```python
from build123d import *

# Parameters (mm, degrees)
F1_DEPTH       = 12.7
F25_DEPTH      = 38.1
F3_D           = 3.175
F3_DEPTH       = 63.5
F3_CBORE_D     = 12.7
F3_CBORE_DEPTH = 6.35
F3_TIP         = 0.9538662327
F5_D           = 3.175
F5_DEPTH       = 63.5
F5_CBORE_D     = 12.7
F5_CBORE_DEPTH = 6.35
F5_TIP         = 0.9538662327
F7_D           = 3.175
F7_DEPTH       = 63.5
F7_TIP         = 0.9538662327
F9_D           = 3.175
F9_DEPTH       = 63.5
F9_TIP         = 0.9538662327
F10_W          = 330.2
F10_H          = 25.4
F11_DEPTH      = 6.35
F12_W          = 426.9362986088
F12_H          = 25.4
F13_DEPTH      = 6.35
F14_W          = 25.4
F14_H          = 558.8
F15_DEPTH      = 3.175
F16_W          = 25.4
F16_H          = 558.8
F17_DEPTH      = 3.175
F19_W          = 12.7
F19_H          = 25.4
F20_DEPTH      = 25.4
F18_W          = 165.1
F18_H          = 25.4
F21_DEPTH      = 3.175
F22_W          = 165.1
F22_H          = 25.4
F23_DEPTH      = 3.175


with BuildPart() as f1:
    # F0 (on Front) → F1 (new body, symmetric)
    with BuildSketch(Plane.XZ):
        with BuildLine():
            Line((165.1, 1828.8), (0, 1828.8))
            Line((0, 1828.8), (-165.1, 1828.8))
            Line((-165.1, 1828.8), (-165.1, 685.8))
            ThreePointArc((-165.1, 685.8), (-187.4175900274, 340.0309838924), (-254, 0))
            Line((-254, 0), (0, 0))
            Line((0, 0), (254, 0))
            ThreePointArc((254, 0), (187.4175900273, 340.0309838924), (165.1, 685.8))
            Line((165.1, 685.8), (165.1, 1828.8))
        make_face()
    extrude(amount=F1_DEPTH, both=True)

    # F24 (on face) → F25 (cut)
    with BuildSketch(Plane.XZ.offset(12.7)):
        Polygon((-12.7, 558.8), (0, 558.8), (12.7, 558.8), (12.7, 1828.8), (0, 1828.8), (-12.7, 1828.8), align=None)
    extrude(amount=-F25_DEPTH, mode=Mode.SUBTRACT)

    # F3
    with Locations(Plane.XZ.offset(12.7)):
        with Locations((-88.9, 1371.6), (88.9, 1371.6)):
            CounterBoreHole(F3_D / 2, F3_CBORE_D / 2, F3_CBORE_DEPTH, depth=F3_DEPTH)
            with Locations((0, 0, -(F3_DEPTH + F3_TIP / 2))):  # 118° drill point
                Cone(0, F3_D / 2, F3_TIP, mode=Mode.SUBTRACT)

    # F5
    with Locations(Plane(origin=(0, 12.7, 0), x_dir=(-1, 0, 0), z_dir=(0, 1, 0))):
        with Locations((-88.9, 457.2), (88.9, 457.2)):
            CounterBoreHole(F5_D / 2, F5_CBORE_D / 2, F5_CBORE_DEPTH, depth=F5_DEPTH)
            with Locations((0, 0, -(F5_DEPTH + F5_TIP / 2))):  # 118° drill point
                Cone(0, F5_D / 2, F5_TIP, mode=Mode.SUBTRACT)

    # F7
    with Locations(Plane.XY.offset(1828.8)):
        with Locations((-127, 0), (127, 0)):
            Hole(F7_D / 2, depth=F7_DEPTH)
            with Locations((0, 0, -(F7_DEPTH + F7_TIP / 2))):  # 118° drill point
                Cone(0, F7_D / 2, F7_TIP, mode=Mode.SUBTRACT)

    # F9
    with Locations(Plane(origin=(0, 0, 0), x_dir=(1, 0, 0), z_dir=(0, 0, -1))):
        with Locations((-190.5, 0), (190.5, 0)):
            Hole(F9_D / 2, depth=F9_DEPTH)
            with Locations((0, 0, -(F9_DEPTH + F9_TIP / 2))):  # 118° drill point
                Cone(0, F9_D / 2, F9_TIP, mode=Mode.SUBTRACT)

    # F10 (on face) → F11 (cut)
    with BuildSketch(Plane(origin=(0, 12.7, 0), x_dir=(-1, 0, 0), z_dir=(0, 1, 0))):
        with Locations((0, 1371.6)):
            Rectangle(F10_W, F10_H)
    extrude(amount=-F11_DEPTH, mode=Mode.SUBTRACT)

    # F12 (on face) → F13 (cut)
    with BuildSketch(Plane.XZ.offset(12.7)):
        with Locations((0, 457.2)):
            Rectangle(F12_W, F12_H)
    extrude(amount=-F13_DEPTH, mode=Mode.SUBTRACT)

    # F14 (on face) → F15 (cut)
    with BuildSketch(Plane(origin=(0, 12.7, 0), x_dir=(-1, 0, 0), z_dir=(0, 1, 0))):
        with Locations((0, 279.4)):
            Rectangle(F14_W, F14_H)
    extrude(amount=-F15_DEPTH, mode=Mode.SUBTRACT)

    # F16 (on face) → F17 (cut)
    with BuildSketch(Plane.XZ.offset(12.7)):
        with Locations((0, 279.4)):
            Rectangle(F16_W, F16_H)
    extrude(amount=-F17_DEPTH, mode=Mode.SUBTRACT)

    # F19 (on face) → F20 (cut)
    with BuildSketch(Plane.XZ.offset(12.7)):
        with Locations((165.1, 914.4)):
            Rectangle(F19_W, F19_H)
    extrude(amount=-F20_DEPTH, mode=Mode.SUBTRACT)

    # F18 (on face) → F21 (cut)
    with BuildSketch(Plane.XZ.offset(12.7)):
        with Locations((82.55, 914.4)):
            Rectangle(F18_W, F18_H)
    extrude(amount=-F21_DEPTH, mode=Mode.SUBTRACT)

    # F22 (on face) → F23 (cut)
    with BuildSketch(Plane(origin=(0, 12.7, 0), x_dir=(-1, 0, 0), z_dir=(0, 1, 0))):
        with Locations((-82.55, 914.4)):
            Rectangle(F22_W, F22_H)
    extrude(amount=-F23_DEPTH, mode=Mode.SUBTRACT)


solid = f1.part
```
The listing builds one solid part. Answer for the finished solid, in the listing's coordinates (mm). Give positions to 0.01 mm unless a question says otherwise; leave off trailing zeros. Write each loop counter-clockwise with the first axis right and the second up, starting at its lowest first coordinate (ties: lowest second). Pieces come first, ordered by that corner, then holes. Notation, with made-up numbers: (-27, 36.5) -> (-16, 36.5) arc R20 ccw to (-16, 75.5) -> close; hole circle Ø10 at (-34.5, 13). An arc over 180 degrees is marked (long way). Write item = value, one per line. Start each with the question number.
1) Each of these flat-tipped pins is pushed along its axis until it touches: pin 1 (6 mm diameter, centred on y = -5.5, z = 1001.5, fed in from -X); pin 2 (6.5 mm diameter, centred on x = -89, z = 460, fed in from +Y); pin 3 (7.5 mm diameter, centred on y = 6, z = 1364, fed in from +X). Where does it stop, or does it pass through?
2) The part is cut by section A-A, the plane z = 980. Determine the outline of the cut face in (x, y), and give its area (3 significant figures).
3) The part is cut by section B-B, the plane z = 178. Determine the outline of the cut face in (x, y) (3 decimals), and give its area (3 significant figures).
4) Straight lines are drawn through the part: line 1 along Z through (x, y) = (88.9, 9.25); line 2 along X through (y, z) = (0, 1809.5); line 3 along X through (y, z) = (-9, 1371.6). For each, find the intervals that lie inside material, in ascending order.
Solutions:
q1.pin_1 = -165.1
q1.pin_2 = 6.35
q1.pin_3 = 165.1
q2.outline = (-165.1, -12.7) -> (-12.7, -12.7) -> (-12.7, 12.7) -> (-165.1, 12.7) -> close; (12.7, -12.7) -> (165.1, -12.7) -> (165.1, 12.7) -> (12.7, 12.7) -> close
q2.area = 7,740 mm²
q3.outline = (-213.47, -12.7) -> (-12.7, -12.7) -> (-12.7, -9.525) -> (12.7, -9.525) -> (12.7, -12.7) -> (213.47, -12.7) -> (213.47, 12.7) -> (12.7, 12.7) -> (12.7, 9.525) -> (-12.7, 9.525) -> (-12.7, 12.7) -> (-213.47, 12.7) -> close
q3.area = 10,700 mm²
q4.line_1 = 0 to 450.85, 463.55 to 1358.9, 1384.3 to 1828.8
q4.line_2 = -165.1 to -128.59, -125.41 to -12.7, 12.7 to 125.41, 128.59 to 165.1
q4.line_3 = -165.1 to -95.25, -82.55 to -12.7, 12.7 to 82.55, 95.25 to 165.1
